For this review, take the finished solid that the model builds, in its own axes (mm). A direction names the side the tool comes from. Give positions to 0.01 mm unless a question says otherwise; leave off trailing zeros. Order: outer loops, then holes, each group sorted by start corner. A loop starts at its lowest first (then second) coordinate and runs counter-clockwise, first axis right, second up.
from build123d import *

# Parameters (mm, degrees)
SKETCH1_R           = 5
SKETCH1_R_2         = 9.017
BOSS_EXTRUDE1_DEPTH = 3.175
BOSS_EXTRUDE2_START = -3.175
SKETCH1_3_R         = 5
BOSS_EXTRUDE2_DEPTH = 6.35
CUT_EXTRUDE1_DEPTH  = 1.3


with BuildPart() as part:
    # Sketch1 → Boss-Extrude1 (new body)
    with BuildSketch(Plane(origin=(0, 0, 0), x_dir=(1, 0, 0), z_dir=(0, 1, 0))):
        with BuildLine():
            Line((-39.315149004, 26.587226943), (-25.231781425, 7.554111896))
            ThreePointArc((-25.231781425, 7.554111896), (-22.740865295, 0), (-25.231781425, -7.554111896))
            Line((-25.231781425, -7.554111896), (-39.315149004, -26.587226943))
            ThreePointArc((-39.315149004, -26.587226943), (-38.434652948, -38.434652948), (-26.587226943, -39.315149004))
            Line((-26.587226943, -39.315149004), (-7.554111896, -25.231781425))
            ThreePointArc((-7.554111896, -25.231781425), (0, -22.740865295), (7.554111896, -25.231781425))
            Line((7.554111896, -25.231781425), (26.587226943, -39.315149004))
            ThreePointArc((26.587226943, -39.315149004), (38.434652948, -38.434652948), (39.315149004, -26.587226943))
            Line((39.315149004, -26.587226943), (25.231781425, -7.554111896))
            ThreePointArc((25.231781425, -7.554111896), (22.740865295, 0), (25.231781425, 7.554111896))
            Line((25.231781425, 7.554111896), (39.315149004, 26.587226943))
            ThreePointArc((39.315149004, 26.587226943), (38.434652948, 38.434652948), (26.587226943, 39.315149004))
            Line((26.587226943, 39.315149004), (7.554111896, 25.231781425))
            ThreePointArc((7.554111896, 25.231781425), (0, 22.740865295), (-7.554111896, 25.231781425))
            Line((-7.554111896, 25.231781425), (-26.587226943, 39.315149004))
            ThreePointArc((-26.587226943, 39.315149004), (-38.434652948, 38.434652948), (-39.315149004, 26.587226943))
        make_face()
        with Locations(Location((-32, -32, 0), (0, 0, 270))):
            Circle(SKETCH1_R, mode=Mode.SUBTRACT)
        with Locations(Location((32, -32, 0), (0, 0, 270))):
            Circle(SKETCH1_R, mode=Mode.SUBTRACT)
        Polygon((-19.642190111, 1.190625), (-19.642190111, 0.396875), (-16.467190111, 0.396875), (-16.467190111, -0.396875), (-19.642190111, -0.396875), (-19.642190111, -1.190625), (-21.704413103, 0), align=None, mode=Mode.SUBTRACT)
        with Locations(Location((-1.27, 0, 0), (0, 0, 270))):
            Circle(SKETCH1_R_2, mode=Mode.SUBTRACT)
        with Locations(Location((-32, 32, 0), (0, 0, 270))):
            Circle(SKETCH1_R, mode=Mode.SUBTRACT)
        with Locations(Location((32, 32, 0), (0, 0, 270))):
            Circle(SKETCH1_R, mode=Mode.SUBTRACT)
    extrude(amount=BOSS_EXTRUDE1_DEPTH)

    # Sketch1<3> → Boss-Extrude2 (add)
    with BuildSketch(Plane(origin=(0, 0, 0), x_dir=(1, 0, 0), z_dir=(0, 1, 0)).offset(BOSS_EXTRUDE2_START)):
        with Locations(Location((-32, 32, 0), (0, 0, 270))):
            Circle(SKETCH1_3_R)
        with Locations(Location((32, -32, 0), (0, 0, 270))):
            Circle(SKETCH1_3_R)
        with Locations(Location((32, 32, 0), (0, 0, 270))):
            Circle(SKETCH1_3_R)
        with Locations(Location((-32, -32, 0), (0, 0, 270))):
            Circle(SKETCH1_3_R)
    extrude(amount=BOSS_EXTRUDE2_DEPTH)

    # Sketch2 → Cut-Extrude1 (cut)
    with BuildSketch(Plane.XZ):
        Polygon((-6.462290551, -24.423898886), (-24.423898886, -6.462290551), (-33.589527929, -18.849276199), (-18.849276199, -33.589527929), align=None)
        Polygon((-33.589527929, 18.849276199), (-18.849276199, 33.589527929), (-6.462290551, 24.423898886), (-24.423898886, 6.462290551), align=None)
        Polygon((24.423898886, 6.462290551), (33.589527929, 18.849276199), (18.849276199, 33.589527929), (6.462290551, 24.423898886), align=None)
        Polygon((33.589527929, -18.849276199), (18.849276199, -33.589527929), (6.462290551, -24.423898886), (24.423898886, -6.462290551), align=None)
    extrude(amount=-CUT_EXTRUDE1_DEPTH, mode=Mode.SUBTRACT)


solid = part.part
1) We need section C-C on z = -15. Give the boundary of the cut face in (x, y) (3 decimals).
Answer sheet:
outline: (-30.741, 1.3) - (-15.886, 1.3) - (-15.886, 0) - (15.886, 0) - (15.886, 1.3) - (30.741, 1.3) - (30.741, 3.175) - (-30.741, 3.175) - close
2) Draft analysis for pull direction X (two halves, no side actions). For faces 1 (the face through (33.94, 1.92, 19.32)), 2 (the face through (11, 0, 0)), 3 (the face through (19.05, 1.92, 33.74)), state which applies: +X half, -X half, draft (parallel to the pull), parting line (faces both ways), or undercut.
Answer sheet:
face 1: +X half
face 2: draft
face 3: undercut
3) We need section B-B on y = -2. Give the boundary of the cut face in (x, z), then the cut area to 3 significant figures.
Answer sheet:
outline: circle Ø10 at (-32, -32); circle Ø10 at (-32, 32); circle Ø10 at (32, -32); circle Ø10 at (32, 32)
area: 314 mm2
4) We need section A-A on x = -1.27. Give the boundary of the cut face in (y, z) (3 decimals), then the cut area to 3 significant figures.
Answer sheet:
outline: (0, -22.805) - (3.175, -22.805) - (3.175, -9.017) - (0, -9.017) - close; (0, 9.017) - (3.175, 9.017) - (3.175, 22.805) - (0, 22.805) - close
area: 87.6 mm2
5) Clearance check with flat-ended pins moving along their axes: pin 1 (2 mm diameter, centred on x = -15.5, z = 28, fed in from -Y); pin 2 (20.5 mm diameter, centred on x = -1.27, z = 0, fed in from -Y); pin 3 (1 mm diameter, centred on y = 2.5, z = -11.5, fed in from -X). State where each tip first meets the part, or that it passes through.
Answer sheet:
pin 1: stops at y = 1.3
pin 2: stops at y = 0
pin 3: stops at x = -28.52
6) Tool access review of faces 4 (the face through (38.305, 1.565, 38.562)), 5 (the face through (-19.32, 1.92, 33.94)), 6 (the face through (-15.317, 0.641, -15.569)): name each direction out of +Z, -Z, +X, -X, +Y, -Y from which nothing blocks a thin tool from reaching the whole face with its end or side.
Answer sheet:
face 4: +Y, -Y
face 5: +Z, +Y, -Y
face 6: -Y
7) We need section D-D on x = 32. Give the boundary of the cut face in (y, z) (3 decimals), then the cut area to 3 significant figures.
Answer sheet:
outline: (-3.175, -37) - (0, -37) - (0, -41.1) - (3.175, -41.1) - (3.175, -16.701) - (1.3, -16.701) - (1.3, -20.439) - (0, -20.439) - (0, -27) - (-3.175, -27) - close; (-3.175, 27) - (0, 27) - (0, 20.439) - (1.3, 20.439) - (1.3, 16.701) - (3.175, 16.701) - (3.175, 41.1) - (0, 41.1) - (0, 37) - (-3.175, 37) - close
area: 209 mm2
8) To check wall thickness, follow line 1 (X direction, y = -2.25, z = -32); line 2 (X direction, y = -2, z = -34.5); line 3 (Y direction, x = 32.5, z = 23) (3 decimals). State the ranges of each line that lie inside material, in increasing order.
Answer sheet:
line 1: x = -37 to -27, 27 to 37
line 2: x = -36.33 to -27.67, 27.67 to 36.33
line 3: y = 0 to 3.175
